Autodesk Inventor part; units mm, degrees
ref_plane "YZ Plane" through (0, 0, 0) normal (1, 0, 0) x (0, 1, 0)
ref_plane "XZ Plane" through (0, 0, 0) normal (0, 1, 0) x (-1, 0, 0)
ref_plane "XY Plane" through (0, 0, 0) normal (0, 0, 1) x (1, 0, 0)
sketch "Esquisse1" plane through (0, 0, 0) normal (0, 1, 0) x (-1, 0, 0)
  circle A0 centre (0, 0) radius 12.5
  dimension "d0" = 25
extrude "Extrusion1" add sketch "Esquisse1" along normal blind 5
sketch "Esquisse3" plane through (0, 0, 0) normal (0, -1, 0) x (1, 0, 0)
  line L0 (-3.5, 0.35) -> (3.5, 0.35)
  line L1 (3.5, 0.35) -> (3.5, -0.35)
  line L2 (3.5, -0.35) -> (-3.5, -0.35)
  line L3 (-3.5, -0.35) -> (-3.5, 0.35)
  line L4 (-3.5, 0.35) -> (3.5, -0.35) construction
  line L5 (3.5, 0.35) -> (-3.5, -0.35) construction
  circle A0 centre (0, 0) radius 3.5
  circle A1 centre (0, 0) radius 7.5
  point P0 (3.4825, 0.35)
  point P1 (-3.4825, 0.35)
  point P2 (3.4825, -0.35)
  point P3 (-3.4825, -0.35)
  dimension "d12" = 0.7
  dimension "d14" = 7
  dimension "d15" = 4
extrude "Extrusion2" add sketch "Esquisse3" along normal blind 7 contours L0 A0 L3 | L0 A0 L2 | A0 L2 L3 | L0 L1 A0 | L1 L2 A0 | A1
ref_plane "Plan de construction1" through (0, 10, 0) normal (0, 1, 0) x (1, 0, 0)
sketch "Esquisse4" plane through (0, 10, 0) normal (0, 1, 0) x (1, 0, 0)
  line L0 (0, 0) -> (0, 22.3046) construction
  line L1 (-26.1226, 0) -> (0, 0) construction
  line L2 (-3.4825, 0.35) -> (3.4825, 0.35)
  arc A0 (2, 5) -> (-12, 5) centre (-5, 5) ccw
  line L3 (-12, 5) -> (2, 5)
  line L4 (-34.5536, 5) -> (31.7867, 5)
  dimension "d19" = 5
  dimension "d20" = 5
  dimension "d21" = 7
revolve "Révolution2" cut sketch "Esquisse4" angle 360 about axis through (-34.5536, 10, -5) along (1, 0, 0)
properties part number "adaptator_potentiometre_test_1"
The listing builds one solid part. Answer for the finished solid, in the listing's coordinates (mm). A direction names the side the tool comes from. Coordinates: 2 decimals unless noted, no trailing zeros. Write each loop counter-clockwise with the first axis right and the second up, starting at its lowest first coordinate (ties: lowest second). Pieces come first, ordered by that corner, then holes. Notation, with made-up numbers: (-8.5, 45.5) -> (16.5, 45.5) arc R20 ccw to (16.5, 66.5) -> close; hole circle Ø7 at (-19, -7.5). An arc over 180 degrees is marked (long way). One line per question, with ' | ' between items.
1. Section B-B (z = -6.5) is taken. Determine the outline of the cut face in (x, y), and give its area (3 significant figures).
Verdict:
outline: (-10.68, 0) -> (-3.74, 0) -> (-3.74, -7) -> (3.74, -7) -> (3.74, 0) -> (10.68, 0) -> (10.68, 5) -> (-0.34, 5) arc R6.84 cw to (-9.66, 5) -> (-10.68, 5) -> close | area: 147 mm^2
2. Section C-C (x = 7) is taken. Determine the outline of the cut face in (y, z).
Verdict:
outline: (-7, -2.69) -> (0, -2.69) -> (0, -10.36) -> (5, -10.36) -> (5, 10.36) -> (0, 10.36) -> (0, 2.69) -> (-7, 2.69) -> close
3. Section D-D (y = 4.25) is taken. Determine the outline of the cut face in (x, z).
Verdict:
outline: circle Ø25 at (0, 0); hole circle Ø7.98 at (-5, -5)
4. For a pull along X with two mould halves and no side action, classify faces 3 (the flat face through (0, -7, 0)), 4 (the cylindrical face through (-7.493, -3.451, -0.33)), 5 (the flat face through (0, -3, -0.35)) as released by +X, released by -X, zero draft, split by the parting line, or undercut.
Verdict:
face 3: zero draft | face 4: split by the parting line | face 5: undercut
5. Straight lines are drawn through the part: line 1 (Z direction, x = 3, y = -0.25); line 2 (Z direction, x = 0.5, y = -1.5); line 3 (Z direction, x = -6.5, y = 4). For each, find the intervals that lie inside material, in ascending order.
Verdict:
line 1: z = -6.87 to -1.8, -0.35 to 0.35, 1.8 to 6.87 | line 2: z = -7.48 to -3.46, -0.35 to 0.35, 3.46 to 7.48 | line 3: z = -10.68 to -8.28, -1.72 to 10.68
6. Section A-A (y = -2.25) is taken. Determine the outline of the cut face in (x, z), and give its area (3 significant figures).
Verdict:
outline: circle Ø15 at (0, 0); hole (-3.48, -0.35) arc R3.5 ccw to (3.48, -0.35) -> close; hole (-3.48, 0.35) -> (3.48, 0.35) arc R3.5 ccw to start | area: 143 mm^2
7. Given pin 1 Ø2.5 at (x, z) = (0.5, 2) entering from -Y; pin 2 Ø5 at (y, z) = (2, -3) entering from +X; pin 3 Ø2 at (x, y) = (-0.5, -3.5) entering from +Z, each flat-ended and moving along its own axis, determine where each tip first touches the part or whether it passes through.
Verdict:
pin 1: stops at y = 0 | pin 2: stops at x = 12.49 | pin 3: stops at z = 7.5
8. Which of the six approach directions +Z, -Z, +X, -X, +Y, -Y give full straight-line access (tool end or side, diameter ignored) to faces 1 (the flat face through (0, -3, 0.35)), 2 (the cylindrical face through (-11.923, 2.465, -3.755))?
Verdict:
face 1: -Y | face 2: +Y, -Y
